Part model, mm, in its own coordinate system. Face numbers are marked on the shaded views. A direction names the side the tool comes from. Give positions to 0.01 mm unless a question says otherwise; leave off trailing zeros. Order: outer loops, then holes, each group sorted by start corner. A loop starts at its lowest first (then second) coordinate and runs counter-clockwise, first axis right, second up. Notation, with made-up numbers: (83.5, 26.25) -> (98.5, 26.25) arc R24 cw to (98.5, 41.25) -> close; hole circle Ø5 at (34.5, 62.5). An arc over 180 degrees is marked (long way). Write item = value, one per line. Start each with the question number.
(1) Flat gauge pins, fed straight in: pin 1 (1.5 mm diameter, centred on x = 28.5, y = 5.5, fed in from -Z); pin 2 (3.5 mm diameter, centred on y = -0.5, z = -5.5, fed in from +X); pin 3 (10 mm diameter, centred on y = 8.5, z = 30, fed in from -X); pin 4 (1.2 mm diameter, centred on y = -0.5, z = 23.5, fed in from -X). Where does each tip first touch, or does it go through?
(2) Probe line 1 along Z through (x, y) = (8, -1.5); line 2 along Y through (x, z) = (48, 4); line 3 along Y through (x, z) = (37.5, 20). List the from-to ranges inside material, lowest first. Write a range as from..to.
(3) Saw through at B-B, the plane x = 0. List the corners of the cut face in (y, z), then the cut area to 3 significant figures.
(4) Saw through at D-D, the plane x = 38. List the corners of the cut face in (y, z).
(5) Which spindle directions (+Z, -Z, +X, -X, +Y, -Y) get a long thin tool onto all of the face, cutting with end or side? Do the marked faces 1, 2, 3 and 4. Say none if no direction does.
(6) Saw through at A-A, the plane z = 2.5. List the corners of the cut face in (x, y), then the cut area to 3 significant figures.
(7) Saw through at C-C, the plane y = 5.5. List the corners of the cut face in (x, z), then the cut area to 3 significant figures.
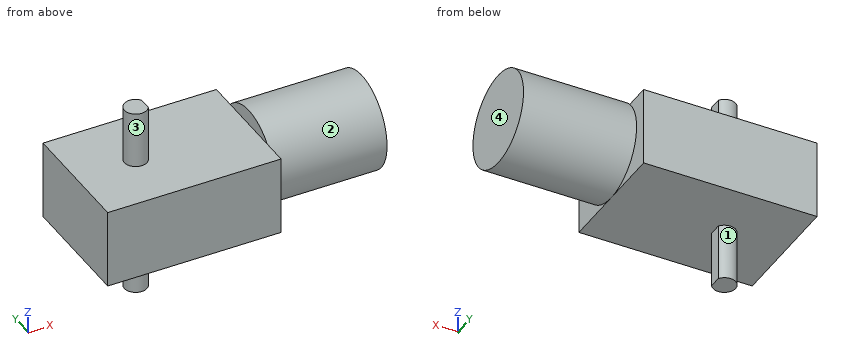
from build123d import *

# Parameters (mm, degrees)
SKETCH_W     = 46
SKETCH_H     = 32
PAD_DEPTH    = 21
SKETCH001_R  = 12.5
PAD001_DEPTH = 30
PAD002_DEPTH = 15
PAD003_DEPTH = 15


with BuildPart() as part:
    # Sketch → Pad (new body)
    with BuildSketch(Plane.XY):
        with Locations((7, 0)):
            Rectangle(SKETCH_W, SKETCH_H)
    extrude(amount=PAD_DEPTH)

    # Sketch001 (on Face2 of Pad) → Pad001 (join)
    with BuildSketch(Plane.YZ.offset(30)):
        with Locations((0, 12.5)):
            Circle(SKETCH001_R)
    extrude(amount=PAD001_DEPTH)

    # Sketch002 (on Face4 of Pad001) → Pad002 (join)
    with BuildSketch(Plane(origin=(0, 0, 0), x_dir=(1, 0, 0), z_dir=(0, 0, -1))):
        with BuildLine():
            ThreePointArc((2.5, 1.658312), (-3, 0), (2.5, -1.658312))
            Line((2.5, 1.658312), (2.5, -1.658312))
        make_face()
    extrude(amount=PAD002_DEPTH)

    # Sketch003 (on Face5 of Pad002) → Pad003 (join)
    with BuildSketch(Plane.XY.offset(21)):
        with BuildLine():
            ThreePointArc((2.5, 1.658312), (-3, 0), (2.5, -1.658312))
            Line((2.5, 1.658312), (2.5, -1.658312))
        make_face()
    extrude(amount=PAD003_DEPTH)


solid = part.part
Results list:
q1.pin_1 = 0
q1.pin_2 = 2.5
q1.pin_3 = through
q1.pin_4 = -3
q2.line_1 = 0..21
q2.line_2 = -9.17..9.17
q2.line_3 = -10..10
q3.outline = (-16, 0) -> (-3, 0) -> (-3, -15) -> (3, -15) -> (3, 0) -> (16, 0) -> (16, 21) -> (3, 21) -> (3, 36) -> (-3, 36) -> (-3, 21) -> (-16, 21) -> close
q3.area = 852 mm^2
q4.outline = circle Ø25 at (0, 12.5)
q5.face_1 = -Z
q5.face_2 = +X
q5.face_3 = +Z
q5.face_4 = +Z, -Z, +X, +Y, -Y
q6.outline = (-16, -16) -> (30, -16) -> (30, -7.5) -> (60, -7.5) -> (60, 7.5) -> (30, 7.5) -> (30, 16) -> (-16, 16) -> close
q6.area = 1,920 mm^2
q7.outline = (-16, 0) -> (30, 0) -> (30, 1.28) -> (60, 1.28) -> (60, 23.72) -> (30, 23.72) -> (30, 21) -> (-16, 21) -> close
q7.area = 1,640 mm^2
